from build123d import *

# Parameters (mm, degrees)
SKETCH1_R           = 20
BOSS_EXTRUDE1_DEPTH = 5
SKETCH2_R           = 3
CUT_EXTRUDE1_DEPTH  = 10
LPATTERN1_COUNT     = 5
LPATTERN1_PITCH     = 10
SKETCH3_R           = 2
CUT_EXTRUDE2_DEPTH  = 116
CUT_EXTRUDE3_START  = -110
SKETCH4_R           = 4.5
CUT_EXTRUDE3_DEPTH  = 9


with BuildPart() as part:
    # Sketch1 → Boss-Extrude1 (new body)
    with BuildSketch(Plane(origin=(0, 0, 0), x_dir=(1, 0, 0), z_dir=(0, 1, 0))):
        with BuildLine():
            Line((-6, -29.393876913), (-6, -150))
            Line((-6, -150), (6, -150))
            Line((6, -150), (6, -29.393876913))
            ThreePointArc((6, -29.393876913), (0, 30), (-6, -29.393876913))
        make_face()
        with Locations(Location((0, 0, 0), (0, 0, 270))):
            Circle(SKETCH1_R, mode=Mode.SUBTRACT)
    extrude(amount=BOSS_EXTRUDE1_DEPTH)

    # Sketch2 → Cut-Extrude1 (cut)
    with BuildSketch(Plane(origin=(0, 5, 0), x_dir=(1, 0, 0), z_dir=(0, 1, 0))):
        with Locations(Location((0, -142, 0), (0, 0, 270))):
            Circle(SKETCH2_R)
    cut_extrude1 = extrude(amount=-CUT_EXTRUDE1_DEPTH, mode=Mode.SUBTRACT)

    # LPattern1: Cut-Extrude1 ×5
    with Locations(*[(0, 0, -i * LPATTERN1_PITCH) for i in range(1, LPATTERN1_COUNT)]):
        add(cut_extrude1, mode=Mode.SUBTRACT)

    # Sketch3 → Cut-Extrude2 (cut)
    with BuildSketch(Plane.XY.offset(150)):
        with Locations((0, 5.5)):
            Circle(SKETCH3_R)
    extrude(amount=-CUT_EXTRUDE2_DEPTH, mode=Mode.SUBTRACT)

    # Sketch4 → Cut-Extrude3 (cut)
    with BuildSketch(Plane.XY.offset(150).offset(CUT_EXTRUDE3_START)):
        with Locations((0, 5.5)):
            Circle(SKETCH4_R)
    extrude(amount=-CUT_EXTRUDE3_DEPTH, mode=Mode.SUBTRACT)


solid = part.part
Design review of the part built by this model. Coordinates are the model's own, in mm. A direction names the side the tool comes from. Round coordinates to 2 decimals unless told otherwise and drop trailing zeros. Loops run counter-clockwise (first coordinate to the right, second up) from the corner with the lowest first, then second, coordinate; pieces in that order, holes last. Notation, with made-up numbers: M 1.5,8.5 L 23.5,8.5 A28 cw 23.5,28.5 Z; hole C 80,3 d2. An arc over 180 degrees is marked long. Answer as a JSON object with one key per item and string values.
Item 1: Wall thickness on L1, parallel to X at y = 1.9, z = 132; L2, parallel to X at y = 1.5, z = 78; L3, parallel to X at y = 3.15, z = -9: over which ranges is each line inside the solid? List them lowest first. Write a range as from..to.
Answer sheet:
{"L1": "x = -6..-3, 3..6", "L2": "x = -6..6", "L3": "x = -28.62..-17.86, 17.86..28.62"}
Item 2: Clearance check with flat-ended pins moving along their axes: P1, Ø2.5, axis at y = 3, z = 93, coming from the +X side; P2, Ø1.2, axis at x = 0.5, y = 3.5, coming from the -Z side; P3, Ø2, axis at x = 20.5, y = 2.5, coming from the +Z side; P4, Ø5.5, axis at x = 0, z = 132, coming from the -Y side. State where each tip first meets the part, or that it passes through.
Answer sheet:
{"P1": "stops at x = 6", "P2": "stops at z = -30", "P3": "stops at z = 22.8", "P4": "passes through"}
Item 3: The part is to be moulded in two halves that separate along Z. For faces 6 (the cylindrical face through (1.235, 2.465, -29.975)), 7 (the flat face through (0, 5, 26)), 8 (the cylindrical face through (3, 3, 122)), say which applies: pulls with the +Z half, pulls with the -Z half, needs draft (parallel to the pull), parting line crosses it, or undercut.
Answer sheet:
{"face 6": "parting line crosses it", "face 7": "needs draft", "face 8": "undercut"}
Item 4: We need section C-C on y = 1.9. Give the boundary of the cut face in (x, z), and give its area (3 significant figures).
Answer sheet:
{"outline": "M -6,29.39 A30 ccw long 6,29.39 L 6,150 L -6,150 Z; hole C 0,0 d40; hole C 0,102 d6; hole C 0,112 d6; hole C 0,122 d6; hole C 0,132 d6; hole C 0,142 d6; hole M -2.7,31 L 2.7,31 L 2.7,40 L -2.7,40 Z", "area": "2,820 mm^2"}
Item 5: We need section B-B on x = 8.5. Give the boundary of the cut face in (y, z).
Answer sheet:
{"outline": "M 0,-28.77 L 5,-28.77 L 5,-18.1 L 0,-18.1 Z; M 0,18.1 L 5,18.1 L 5,28.77 L 0,28.77 Z"}
Item 6: We need section D-D on z = 86.5. Give the boundary of the cut face in (x, y), and give its area (3 significant figures).
Answer sheet:
{"outline": "M -6,0 L 6,0 L 6,5 L 1.94,5 A2 cw -1.94,5 L -6,5 Z", "area": "55.7 mm^2"}
Item 7: Machinability: for faces 1 (the flat face through (-6, 2, 89)), 2 (the cylindrical face through (-19.524, 2.465, -4.336)), 3 (the flat face through (6, 2, 91)), 4 (the cylindrical face through (0, 1, 36)), 5 (the cylindrical face through (0, 3.5, 107)), which of the approach directions +Z, -Z, +X, -X, +Y, -Y give a long, thin tool a straight path to every point of the face, cutting with its end or side? Answer none if there is none.
Answer sheet:
{"face 1": "+Z, -X, +Y, -Y", "face 2": "+Y, -Y", "face 3": "+Z, +X, +Y, -Y", "face 4": "+Y", "face 5": "+Z, +Y"}
Item 8: We need section A-A on z = 0. Give the boundary of the cut face in (x, y), and give its area (4 significant figures).
Answer sheet:
{"outline": "M -30,0 L -20,0 L -20,5 L -30,5 Z; M 20,0 L 30,0 L 30,5 L 20,5 Z", "area": "100.0 mm^2"}
